from build123d import *

# Parameters (mm, degrees)
F0_R     = 0.75
F1_DEPTH = 2.5
F2_R     = 4.4
F2_R_2   = 2.7
F3_DEPTH = 3
F4_R     = 1.425
F5_DEPTH = 25
F6_DEPTH = 0.6


with BuildPart() as f1:
    # F0 (on Top) → F1 (new body)
    with BuildSketch(Plane.XY):
        with BuildLine():
            ThreePointArc((6.62495283, 4), (6.1790882982, 4.1048995479), (5.8267657421, 4.3975903614))
            ThreePointArc((5.8267657421, 4.3975903614), (5.1832727919, 5.1403971796), (4.4458365341, 5.7900377816))
            ThreePointArc((4.4458365341, 5.7900377816), (4.1579107845, 6.1410503979), (4.0548552374, 6.5831936421))
            Line((4.0548552374, 6.5831936421), (4.0548552374, 8.6677777952))
            ThreePointArc((4.0548552374, 8.6677777952), (4.0350683201, 8.865723021), (3.9764906125, 9.0558347952))
            Line((3.9764906125, 9.0558347952), (0.2764906125, 17.8433347952))
            ThreePointArc((0.2764906125, 17.8433347952), (0, 18.0269176952), (-0.2764906125, 17.8433347952))
            Line((-0.2764906125, 17.8433347952), (-3.9216353751, 9.186115984))
            ThreePointArc((-3.9216353751, 9.186115984), (-3.9802130827, 8.9960042098), (-4, 8.798058984))
            Line((-4, 8.798058984), (-4, 6.62495283))
            ThreePointArc((-4, 6.62495283), (-4.1048995479, 6.1790882982), (-4.3975903614, 5.8267657421))
            ThreePointArc((-4.3975903614, 5.8267657421), (-5.1618795027, 5.1618795027), (-5.8267657421, 4.3975903614))
            ThreePointArc((-5.8267657421, 4.3975903614), (-6.1790882982, 4.1048995479), (-6.62495283, 4))
            Line((-6.62495283, 4), (-8.798058984, 4))
            ThreePointArc((-8.798058984, 4), (-8.9960042098, 3.9802130827), (-9.186115984, 3.9216353751))
            Line((-9.186115984, 3.9216353751), (-17.8433347952, 0.2764906125))
            ThreePointArc((-17.8433347952, 0.2764906125), (-18.0269176952, 0), (-17.8433347952, -0.2764906125))
            Line((-17.8433347952, -0.2764906125), (-9.186115984, -3.9216353751))
            ThreePointArc((-9.186115984, -3.9216353751), (-8.9960042098, -3.9802130827), (-8.798058984, -4))
            Line((-8.798058984, -4), (-6.62495283, -4))
            ThreePointArc((-6.62495283, -4), (-6.1790882982, -4.1048995479), (-5.8267657421, -4.3975903614))
            ThreePointArc((-5.8267657421, -4.3975903614), (-5.1618795027, -5.1618795027), (-4.3975903614, -5.8267657421))
            ThreePointArc((-4.3975903614, -5.8267657421), (-4.1048995479, -6.1790882982), (-4, -6.62495283))
            Line((-4, -6.62495283), (-4, -8.798058984))
            ThreePointArc((-4, -8.798058984), (-3.9802130827, -8.9960042098), (-3.9216353751, -9.186115984))
            Line((-3.9216353751, -9.186115984), (-0.2764906125, -17.8433347952))
            ThreePointArc((-0.2764906125, -17.8433347952), (0, -18.0269176952), (0.2764906125, -17.8433347952))
            Line((0.2764906125, -17.8433347952), (3.9764906125, -9.0558347952))
            ThreePointArc((3.9764906125, -9.0558347952), (4.0350683201, -8.865723021), (4.0548552374, -8.6677777952))
            Line((4.0548552374, -8.6677777952), (4.0548552374, -6.5831936421))
            ThreePointArc((4.0548552374, -6.5831936421), (4.1579107845, -6.1410503979), (4.4458365341, -5.7900377816))
            ThreePointArc((4.4458365341, -5.7900377816), (5.1832727919, -5.1403971796), (5.8267657421, -4.3975903614))
            ThreePointArc((5.8267657421, -4.3975903614), (6.1790882982, -4.1048995479), (6.62495283, -4))
            Line((6.62495283, -4), (8.798058984, -4))
            ThreePointArc((8.798058984, -4), (8.9960042098, -3.9802130827), (9.186115984, -3.9216353751))
            Line((9.186115984, -3.9216353751), (17.8433347952, -0.2764906125))
            ThreePointArc((17.8433347952, -0.2764906125), (18.0269176952, 0), (17.8433347952, 0.2764906125))
            Line((17.8433347952, 0.2764906125), (9.186115984, 3.9216353751))
            ThreePointArc((9.186115984, 3.9216353751), (8.9960042098, 3.9802130827), (8.798058984, 4))
            Line((8.798058984, 4), (6.62495283, 4))
        make_face()
        with Locations((0, -15.6)):
            Circle(F0_R, mode=Mode.SUBTRACT)
        with Locations((0, -12.8)):
            Circle(F0_R, mode=Mode.SUBTRACT)
        with Locations((0, -10)):
            Circle(F0_R, mode=Mode.SUBTRACT)
        with Locations((0, -7.2)):
            Circle(F0_R, mode=Mode.SUBTRACT)
        with Locations((-15.6, 0)):
            Circle(F0_R, mode=Mode.SUBTRACT)
        with Locations((-12.8, 0)):
            Circle(F0_R, mode=Mode.SUBTRACT)
        with Locations((-10, 0)):
            Circle(F0_R, mode=Mode.SUBTRACT)
        with Locations((-7.2, 0)):
            Circle(F0_R, mode=Mode.SUBTRACT)
        with Locations((7.2, 0)):
            Circle(F0_R, mode=Mode.SUBTRACT)
        with Locations((0, 7.2)):
            Circle(F0_R, mode=Mode.SUBTRACT)
        with Locations((10, 0)):
            Circle(F0_R, mode=Mode.SUBTRACT)
        with Locations((12.8, 0)):
            Circle(F0_R, mode=Mode.SUBTRACT)
        with Locations((15.6, 0)):
            Circle(F0_R, mode=Mode.SUBTRACT)
        with Locations((0, 10)):
            Circle(F0_R, mode=Mode.SUBTRACT)
        with Locations((0, 12.8)):
            Circle(F0_R, mode=Mode.SUBTRACT)
        with Locations((0, 15.6)):
            Circle(F0_R, mode=Mode.SUBTRACT)
    extrude(amount=F1_DEPTH)

    # F2 (on face) → F3 (join)
    with BuildSketch(Plane(origin=(0, 0, 0), x_dir=(1, 0, 0), z_dir=(0, 0, -1))):
        Circle(F2_R)
        Circle(F2_R_2, mode=Mode.SUBTRACT)
    extrude(amount=F3_DEPTH)

    # F4 (on face) → F5 (cut)
    with BuildSketch(Plane(origin=(0, 0, 0), x_dir=(1, 0, 0), z_dir=(0, 0, -1))):
        Circle(F4_R)
    extrude(amount=-F5_DEPTH, mode=Mode.SUBTRACT)

    # F6 (cut): a face of the model
    f6_faces = [f1.faces().sort_by_distance(p)[0] for p in [
        (-2.6236324676, 0, 0),
    ]]
    extrude(f6_faces, amount=-F6_DEPTH, mode=Mode.SUBTRACT)


solid = f1.part
The model under review builds one solid part; all positions refer to its coordinate system, in mm. A direction names the side the tool comes from. Give positions to 0.01 mm unless a question says otherwise; leave off trailing zeros. Loops run counter-clockwise (first coordinate to the right, second up) from the corner with the lowest first, then second, coordinate; pieces in that order, holes last. Notation, with made-up numbers: (79.5, 46) -> (113.5, 46) arc R11 cw to (113.5, 56) -> close; hole circle Ø9 at (76, 38). An arc over 180 degrees is marked (long way). Answer as a JSON object with one key per item and string values. Group by question number.
Q1. Insertion check: pin 1 (1.5 mm diameter, centred on x = 1.5, y = -8.5, fed in from -Z); pin 2 (1.5 mm diameter, centred on x = 0.5, z = -1.5, fed in from -Y); pin 3 (1.1 mm diameter, centred on y = 7.5, z = 1, fed in from -X). Each pin has a flat end and moves straight along its axis. Give the tip position at first contact, or say it passes through.
Q2. Tool access review of faces 5 (the cylindrical face through (-0.098, -6.456, 1.232)), 6 (the flat face through (1.2, -1.2, 0.6)): name each direction out of +Z, -Z, +X, -X, +Y, -Y from which nothing blocks a thin tool from reaching the whole face with its end or side.
Q3. Take a section at C-C (y = -2). Write out the cut boundary in (x, z).
Q4. Wall thickness on line 1 along Y through (x, z) = (-7.2, 1.45); line 2 along Z through (x, y) = (1, 15); line 3 along Y through (x, z) = (15.6, 1.2): over which ranges is each line inside the solid? List them lowest first.
Q5. Draft analysis for pull direction X (two halves, no side actions). For faces 1 (the cylindrical face through (16.315, 0.225, 1.232)), 2 (the flat face through (3, -4, 0)), 3 (the cylindrical face through (5.174, -5.15, 1.232)), 4 (the flat face through (-4, 8, 1)), state which applies: pulls with the +X half, pulls with the -X half, needs draft (parallel to the pull), parting line crosses it, or undercut.
Q6. Take a section at A-A (y = -7.2). Write out the cut boundary in (x, z).
Q7. Take a section at B-B (x = 7.2). Write out the cut boundary in (y, z).
Answer below:
{
 "1": {"pin 1": "stops at z = 0", "pin 2": "stops at y = -4.4", "pin 3": "stops at x = -4"},
 "2": {"face 5": "+Z, -Z", "face 6": "-Z"},
 "3": {"outline": "(-13.75, 0) -> (-3.92, 0) -> (-3.92, -3) -> (-1.81, -3) -> (-1.81, 0.6) -> (1.81, 0.6) -> (1.81, -3) -> (3.92, -3) -> (3.92, 0) -> (13.75, 0) -> (13.75, 2.5) -> (-13.75, 2.5) -> close"},
 "4": {"line 1": "y = -4 to -0.75, 0.75 to 4", "line 2": "z = 0 to 2.5", "line 3": "y = -1.22 to -0.75, 0.75 to 1.22"},
 "5": {"face 1": "undercut", "face 2": "needs draft", "face 3": "pulls with the +X half", "face 4": "pulls with the -X half"},
 "6": {"outline": "(-4, 0) -> (-0.75, 0) -> (-0.75, 2.5) -> (-4, 2.5) -> close; (0.75, 0) -> (4.05, 0) -> (4.05, 2.5) -> (0.75, 2.5) -> close"},
 "7": {"outline": "(-4, 0) -> (-0.75, 0) -> (-0.75, 2.5) -> (-4, 2.5) -> close; (0.75, 0) -> (4, 0) -> (4, 2.5) -> (0.75, 2.5) -> close"}
}
